from build123d import *

# Parameters (mm, degrees)
SKETCH1_R           = 137.941576563
EXTRUDE1_DEPTH      = 3.175
SKETCH2_W           = 19.05
SKETCH2_H           = 25.4
EXTRUDE2_DEPTH      = 4.175
SKETCH3_OUTSIDE_W   = 355.918
SKETCH3_OUTSIDE_H   = 355.918
SKETCH3_OUTSIDE_W_2 = 212.725
SKETCH3_OUTSIDE_H_2 = 133.35
EXTRUDE3_DEPTH      = 4.175
EXTRUDE4_DEPTH      = 3.175


with BuildPart() as part:
    # Sketch1 → Extrude1 (new body)
    with BuildSketch(Plane(origin=(0, 0, 0), x_dir=(1, 0, 0), z_dir=(0, 1, 0))):
        with Locations(Location((0, 0, 0), (0, 0, 270))):  # turned: the seam where the file's is
            Circle(SKETCH1_R)
    extrude(amount=EXTRUDE1_DEPTH)

    # Sketch2 → Extrude2 (cut, through all)
    with BuildSketch(Plane(origin=(0, 3.175, 0), x_dir=(-1, 0, 0), z_dir=(0, 1, 0))):
        with Locations((63.5, -47.625)):
            Rectangle(SKETCH2_W, SKETCH2_H)
        with Locations((63.5, 47.625)):
            Rectangle(SKETCH2_W, SKETCH2_H)
        with Locations((-63.5, 47.625)):
            Rectangle(SKETCH2_W, SKETCH2_H)
        with Locations((-63.5, -47.625)):
            Rectangle(SKETCH2_W, SKETCH2_H)
    extrude(amount=-EXTRUDE2_DEPTH, mode=Mode.SUBTRACT)

    # Sketch3 outside → Extrude3 (cut, through all)
    with BuildSketch(Plane(origin=(0, 3.175, 0), x_dir=(1, 0, 0), z_dir=(0, 1, 0))):
        Rectangle(SKETCH3_OUTSIDE_W, SKETCH3_OUTSIDE_H)
        Rectangle(SKETCH3_OUTSIDE_W_2, SKETCH3_OUTSIDE_H_2, mode=Mode.SUBTRACT)
    extrude(amount=-EXTRUDE3_DEPTH, mode=Mode.SUBTRACT)

    # Sketch4 → Extrude4 (add, through all)
    with BuildSketch(Plane(origin=(0, 3.175, 0), x_dir=(-1, 0, 0), z_dir=(0, 1, 0))):
        with BuildLine():
            Line((-25.4, -66.675), (25.4, -66.675))
            Line((25.4, -66.675), (25.4, -85.725))
            ThreePointArc((25.4, -85.725), (0, -111.125), (-25.4, -85.725))
            Line((-25.4, -85.725), (-25.4, -66.675))
        make_face()
        with BuildLine():
            Line((25.4, 66.675), (25.4, 85.725))
            ThreePointArc((25.4, 85.725), (0, 111.125), (-25.4, 85.725))
            Line((-25.4, 85.725), (-25.4, 66.675))
            Line((-25.4, 66.675), (25.4, 66.675))
        make_face()
    extrude(amount=-EXTRUDE4_DEPTH)


solid = part.part
The listing builds one solid part. Answer for the finished solid, in the listing's coordinates (mm). Round coordinates to 2 decimals unless told otherwise and drop trailing zeros. Loops run counter-clockwise (first coordinate to the right, second up) from the corner with the lowest first, then second, coordinate; pieces in that order, holes last. Notation, with made-up numbers: M 67.25,-37 L 87.25,-37 A5 cw 87.25,-30 Z; hole C 89,24 d5. An arc over 180 degrees is marked long. Return JSON: item names as keys, results as strings.
Q1. Find section D-D, the plane z = 91. Determine the outline of the cut face in (x, y) (3 decimals), plus the area to 3 significant figures.
Results list:
{"outline": "M -24.846,0 L 24.846,0 L 24.846,3.175 L -24.846,3.175 Z", "area": "158 mm2"}
Q2. Find the intervals of material crossed by line 1 along X through (y, z) = (1, 47) (1 decimal); line 2 along Z through (x, y) = (-62, 1.05) (3 decimals); line 3 along Z through (x, y) = (74, 2.65) (3 decimals), in increasing order. Write a range as from..to.
Results list:
{"line 1": "x = -106.4..-73, -54..54, 73..106.4", "line 2": "z = -66.675..-60.325, -34.925..34.925, 60.325..66.675", "line 3": "z = -66.675..66.675"}
Q3. Each of these flat-tipped pins is pushed along its axis until it touches: pin 1 Ø1.6 at (x, y) = (-60, 2.5) entering from -Z (3 decimals); pin 2 Ø1 at (x, y) = (-9.5, 0.5) entering from -Z; pin 3 Ø1 at (y, z) = (2, -76) entering from +X. Where does it stop, or does it pass through?
Results list:
{"pin 1": "stops at z = -66.675", "pin 2": "stops at z = -109.48", "pin 3": "stops at x = 25.4"}
Q4. Find section A-A, the plane x = 69. Determine the outline of the cut face in (y, z) (3 decimals), plus the area to 3 significant figures.
Results list:
{"outline": "M 0,-66.675 L 3.175,-66.675 L 3.175,-60.325 L 0,-60.325 Z; M 0,-34.925 L 3.175,-34.925 L 3.175,34.925 L 0,34.925 Z; M 0,60.325 L 3.175,60.325 L 3.175,66.675 L 0,66.675 Z", "area": "262 mm2"}
Q5. Find section B-B, the plane z = -41.5. Determine the outline of the cut face in (x, y) (1 decimal), plus the area to 3 significant figures.
Results list:
{"outline": "M -106.4,0 L -73,0 L -73,3.2 L -106.4,3.2 Z; M -54,0 L 54,0 L 54,3.2 L -54,3.2 Z; M 73,0 L 106.4,0 L 106.4,3.2 L 73,3.2 Z", "area": "554 mm2"}
Q6. Find section C-C, the plane y = 0.95. Determine the outline of the cut face in (x, z) (1 decimal).
Results list:
{"outline": "M -106.4,-66.7 L -25.4,-66.7 L -25.4,-85.7 A25.4 ccw 25.4,-85.7 L 25.4,-66.7 L 106.4,-66.7 L 106.4,66.7 L 25.4,66.7 L 25.4,85.7 A25.4 ccw -25.4,85.7 L -25.4,66.7 L -106.4,66.7 Z; hole M -73,-60.3 L -54,-60.3 L -54,-34.9 L -73,-34.9 Z; hole M -73,34.9 L -54,34.9 L -54,60.3 L -73,60.3 Z; hole M 54,-60.3 L 73,-60.3 L 73,-34.9 L 54,-34.9 Z; hole M 54,34.9 L 73,34.9 L 73,60.3 L 54,60.3 Z"}
